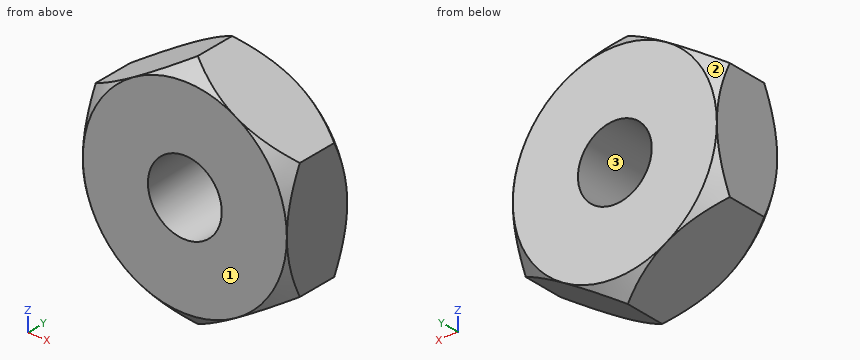
```python
from build123d import *

# Parameters (mm, degrees)
BOSS_EXTRUDE1_DEPTH       = 1.125
F_4_40_TAPPED_HOLE1_D     = 2.2606
F_4_40_TAPPED_HOLE1_DEPTH = 8.87
F_4_40_TAPPED_HOLE1_TIP   = 0.679152758


with BuildPart() as part:
    # Sketch1 → Boss-Extrude1 (new, symmetric)
    with BuildSketch(Plane(origin=(0, 0, 0), x_dir=(1, 0, 0), z_dir=(0, 1, 0))):
        Polygon((0, 3.608439182), (-3.125, 1.804219591), (-3.125, -1.804219591), (0, -3.608439182), (3.125, -1.804219591), (3.125, 1.804219591), align=None)
    extrude(amount=BOSS_EXTRUDE1_DEPTH, both=True)

    # Sketch2 → Cut-Revolve2 (revolve, cut)
    with BuildSketch(Plane.XY):
        Polygon((-4.25, 1.125), (-4.25, 0), (-3.125, 1.125), align=None)
    cut_revolve2 = revolve(axis=Axis((0, 4.25, 0), (0, -1, 0)), mode=Mode.SUBTRACT)

    # Mirror1: Cut-Revolve2 across plane
    add(cut_revolve2.mirror(Plane.ZX), mode=Mode.SUBTRACT)

    # #4-40 Tapped Hole1
    with Locations(Plane(origin=(0, 1.125, 0), x_dir=(1, 0, 0), z_dir=(0, 1, 0))):
        with Locations((0, 0)):
            Hole(F_4_40_TAPPED_HOLE1_D / 2, depth=F_4_40_TAPPED_HOLE1_DEPTH)
            with Locations((0, 0, -(F_4_40_TAPPED_HOLE1_DEPTH + F_4_40_TAPPED_HOLE1_TIP / 2))):  # 118° drill point
                Cone(0, F_4_40_TAPPED_HOLE1_D / 2, F_4_40_TAPPED_HOLE1_TIP, mode=Mode.SUBTRACT)


solid = part.part
```
Work out the finished part from the listing and answer in its coordinate system (mm). Face numbers are marked on the shaded views. Coordinates: 2 decimals unless noted, no trailing zeros. Write each loop counter-clockwise with the first axis right and the second up, starting at its lowest first coordinate (ties: lowest second). Pieces come first, ordered by that corner, then holes.
Q1. A cutting plane is placed at A-A, the plane y = 0.15. Give the vertices of the cut face in (x, z) (3 decimals).
Q2. This flat-tipped pin is pushed along its axis until it touches: pin 1 Ø3.5 at (x, z) = (0, 0) entering from -Y (3 decimals). Where does it stop, or does it pass through?
Q3. Find the intervals of material crossed by line 1 (X direction, y = -0.2, z = 0.5) (3 decimals); line 2 (X direction, y = 0.55, z = -1) (3 decimals); line 3 (Z direction, x = 0, y = 1), in increasing order.
Q4. A cutting plane is placed at B-B, the plane y = -0.95. Give the vertices of the cut face in (x, z) (3 decimals).
Q5. Determine the mould class of the marked faces 1, 2 and 3 for opening direction Z: released by +Z, released by -Z, zero draft, split by the parting line, or undercut.
Q6. A cutting plane is placed at C-C, the plane y = 1. Give the vertices of the cut face in (x, z) (3 decimals).
Findings below:
1. outline: (-3.125, -1.804) - (0, -3.608) - (3.125, -1.804) - (3.125, 1.804) - (0, 3.608) - (-3.125, 1.804) - close; hole circle Ø2.261 at (0, 0)
2. pin 1: stops at y = -1.125
3. line 1: x = -3.125 to -1.014, 1.014 to 3.125
3. line 2: x = -3.125 to -0.527, 0.527 to 3.125
3. line 3: z = -3.25 to -1.13, 1.13 to 3.25
4. outline: (-3.125, -1.06) arc R3.3 ccw to (-2.481, -2.176) - (-0.644, -3.237) arc R3.3 ccw to (0.644, -3.237) - (2.481, -2.176) arc R3.3 ccw to (3.125, -1.06) - (3.125, 1.06) arc R3.3 ccw to (2.481, 2.176) - (0.644, 3.237) arc R3.3 ccw to (-0.644, 3.237) - (-2.481, 2.176) arc R3.3 ccw to (-3.125, 1.06) - close; hole circle Ø2.261 at (0, 0)
5. face 1: zero draft
5. face 2: released by +Z
5. face 3: undercut
6. outline: (-3.125, -0.893) arc R3.25 ccw to (-2.336, -2.26) - (-0.789, -3.153) arc R3.25 ccw to (0.789, -3.153) - (2.336, -2.26) arc R3.25 ccw to (3.125, -0.893) - (3.125, 0.893) arc R3.25 ccw to (2.336, 2.26) - (0.789, 3.153) arc R3.25 ccw to (-0.789, 3.153) - (-2.336, 2.26) arc R3.25 ccw to (-3.125, 0.893) - close; hole circle Ø2.261 at (0, 0)
